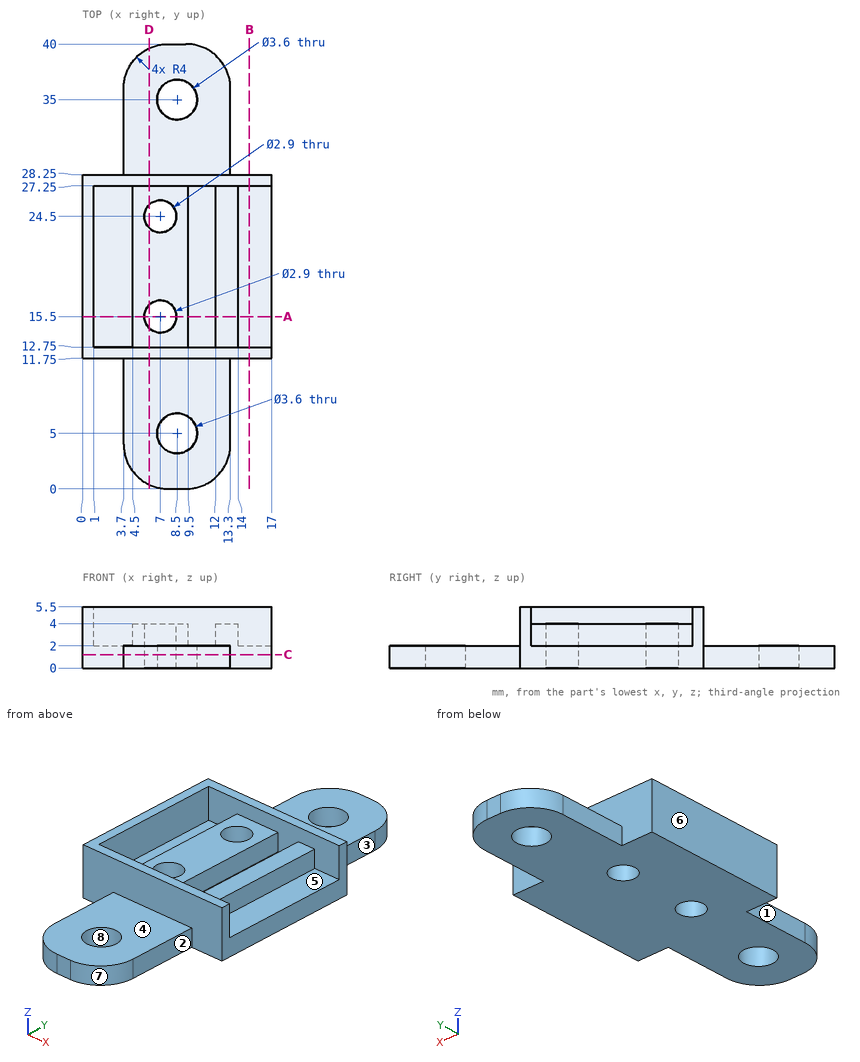
Here's the drawing with two shaded views (mm, measured from the low corner). I have some questions. A direction names the side the tool comes from. Round coordinates to 2 decimals unless told otherwise and drop trailing zeros. Loops run counter-clockwise (first coordinate to the right, second up) from the corner with the lowest first, then second, coordinate; pieces in that order, holes last.
Item 1: Will these pins go through, and if not, where does the flat tip stop? pin 1 Ø0.8 at (x, y) = (11.5, 20.5) entering from +Z; pin 2 Ø3.5 at (x, y) = (7, 15.5) entering from +Z; pin 3 Ø1 at (y, z) = (8, 1) entering from +X.
Item 2: Suppose I cut it at A-A, the plane y = 15.5. Write out the boundary of the cut face in (x, z).
Item 3: Suppose I cut it at C-C, the plane z = 1.2. Write out the boundary of the cut face in (x, y), then the cut area to 3 significant figures.
Item 4: Suppose I cut it at B-B, the plane x = 15. Write out the boundary of the cut face in (y, z), then the cut area to 3 significant figures.
Item 5: Please list where these lines run through material, in increasing order: L1, parallel to Y at x = 8.5, z = 0.9; L2, parallel to X at y = 15.5, z = 2.85; L3, parallel to X at y = 19, z = 2.2.
Item 6: Which directions (+Z, -Z, +X, -X, +Y, -Y) give clear straight access to the entire face, cutting with the end or side of a thin tool? Please do the marked faces 1, 2, 3, 4 and 5.
Item 7: If we mould it in two halves opening along Y, with no side actions, what happens to the marked faces 6, 7 and 8? For each: +Y half, -Y half, draft (parallel to the pull), parting line (faces both ways), or undercut.
Item 8: Suppose I cut it at D-D, the plane x = 6. Write out the boundary of the cut face in (y, z).
Reported:
1. pin 1: stops at z = 2
1. pin 2: stops at z = 4
1. pin 3: stops at x = 13.3
2. outline: (0, 0) - (5.55, 0) - (5.55, 4) - (4.5, 4) - (4.5, 2) - (1, 2) - (1, 5.5) - (0, 5.5) - close; (8.45, 0) - (17, 0) - (17, 2) - (14, 2) - (14, 4) - (12, 4) - (12, 2) - (9.5, 2) - (9.5, 4) - (8.45, 4) - close
3. outline: (0, 11.75) - (3.7, 11.75) - (3.7, 4) arc R4 ccw to (7.7, 0) - (9.3, 0) arc R4 ccw to (13.3, 4) - (13.3, 11.75) - (17, 11.75) - (17, 28.25) - (13.3, 28.25) - (13.3, 36) arc R4 ccw to (9.3, 40) - (7.7, 40) arc R4 ccw to (3.7, 36) - (3.7, 28.25) - (0, 28.25) - close; hole circle Ø2.9 at (7, 15.5); hole circle Ø2.9 at (7, 24.5); hole circle Ø3.6 at (8.5, 5); hole circle Ø3.6 at (8.5, 35)
3. area: 459 mm2
4. outline: (11.75, 0) - (28.25, 0) - (28.25, 5.5) - (27.25, 5.5) - (27.25, 2) - (12.75, 2) - (12.75, 5.5) - (11.75, 5.5) - close
4. area: 40.0 mm2
5. L1: y = 0 to 3.2, 6.8 to 33.2, 36.8 to 40
5. L2: x = 0 to 1, 4.5 to 5.55, 8.45 to 9.5, 12 to 14
5. L3: x = 0 to 1, 4.5 to 9.5, 12 to 14
6. face 1: +Z, -Z, -X, -Y
6. face 2: +Z, -Z, +X, -Y
6. face 3: +Z, -Z, +X, +Y
6. face 4: +Z, +X, -X, -Y
6. face 5: +Z, +X
7. face 6: draft
7. face 7: -Y half
7. face 8: undercut
8. outline: (0.38, 0) - (14.45, 0) - (14.45, 4) - (12.75, 4) - (12.75, 5.5) - (11.75, 5.5) - (11.75, 2) - (0.38, 2) - close; (16.55, 0) - (23.45, 0) - (23.45, 4) - (16.55, 4) - close; (25.55, 0) - (39.62, 0) - (39.62, 2) - (28.25, 2) - (28.25, 5.5) - (27.25, 5.5) - (27.25, 4) - (25.55, 4) - close
